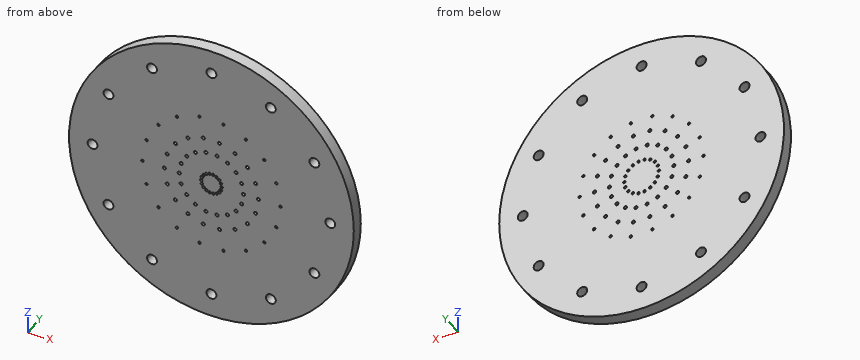
from build123d import *

# Parameters (mm, degrees)
SKETCH1_R           = 73.025
BOSS_EXTRUDE1_DEPTH = 6.35
SKETCH4_R           = 0.59055
CUT_EXTRUDE1_DEPTH  = 50.8475
CUT_EXTRUDE2_START  = -53.3875
SKETCH6_R           = 0.59055
CUT_EXTRUDE2_DEPTH  = 80.524261314
LOX_START           = -7.35
SKETCH7_R           = 0.80645
LOX_HOLES_DEPTH     = 8.35
CIRPATTERN1_COUNT   = 18
SKETCH8_R           = 2.54
CUT_EXTRUDE4_DEPTH  = 7.35
CIRPATTERN2_COUNT   = 12


with BuildPart() as part:
    # Sketch1 → Boss-Extrude1 (new body)
    with BuildSketch(Plane(origin=(0, 0, 0), x_dir=(1, 0, 0), z_dir=(0, 1, 0))):
        Circle(SKETCH1_R)
    extrude(amount=BOSS_EXTRUDE1_DEPTH)

    # Sketch4 → Cut-Extrude1 (cut, through all)
    with BuildSketch(Plane(origin=(-3.917869343, -6.785948759, 0), x_dir=(-0.866025404, 0.5, 0), z_dir=(0.5, 0.866025404, 0))):
        with Locations((-4.52396584, 0)):
            Circle(SKETCH4_R)
    cut_extrude1 = extrude(amount=CUT_EXTRUDE1_DEPTH, mode=Mode.SUBTRACT)

    # Sketch6 → Cut-Extrude2 (cut)
    with BuildSketch(Plane(origin=(5.187869343, -8.985653285, 0), x_dir=(0.866025404, 0.5, 0), z_dir=(0.5, -0.866025404, 0)).offset(CUT_EXTRUDE2_START)):
        with Locations((30.67130657, 0)):
            Circle(SKETCH6_R)
    cut_extrude2 = extrude(amount=CUT_EXTRUDE2_DEPTH, mode=Mode.SUBTRACT)

    # Sketch7 → LOx Holes (cut)
    with BuildSketch(Plane(origin=(0, 6.35, 0), x_dir=(1, 0, 0), z_dir=(0, 1, 0)).offset(LOX_START)):
        with Locations((24.13, 0)):
            Circle(SKETCH7_R)
        with Locations((16.51, 0)):
            Circle(SKETCH7_R)
    lox_holes = extrude(amount=LOX_HOLES_DEPTH, mode=Mode.SUBTRACT)

    # CirPattern1: Cut-Extrude1, Cut-Extrude2, LOx Holes ×18 about axis
    cirpattern1_axis = Axis((0, 0, 0), (0, 1, 0))
    for i in range(1, CIRPATTERN1_COUNT):
        add(cut_extrude1.rotate(cirpattern1_axis, i * 360 / CIRPATTERN1_COUNT), mode=Mode.SUBTRACT)
        add(cut_extrude2.rotate(cirpattern1_axis, i * 360 / CIRPATTERN1_COUNT), mode=Mode.SUBTRACT)
        add(lox_holes.rotate(cirpattern1_axis, i * 360 / CIRPATTERN1_COUNT), mode=Mode.SUBTRACT)

    # Sketch8 → Cut-Extrude4 (cut, through all)
    with BuildSketch(Plane.XZ):
        with Locations((-60.96, 0)):
            Circle(SKETCH8_R)
    cut_extrude4 = extrude(amount=-CUT_EXTRUDE4_DEPTH, mode=Mode.SUBTRACT)

    # CirPattern2: Cut-Extrude4 ×12 about axis
    cirpattern2_axis = Axis((0, 0, 0), (0, 1, 0))
    for i in range(1, CIRPATTERN2_COUNT):
        add(cut_extrude4.rotate(cirpattern2_axis, i * 360 / CIRPATTERN2_COUNT), mode=Mode.SUBTRACT)


solid = part.part
Check sheet for the modelled part. Datum: model origin and axes. Units: mm. Coordinates: 2 decimals unless noted, no trailing zeros. Loops run counter-clockwise (first coordinate to the right, second up) from the corner with the lowest first, then second, coordinate; pieces in that order, holes last. Notation, with made-up numbers: (38, -40) -> (66, -40) arc R9 ccw to (66, -25) -> close; hole circle Ø2 at (-17, 78). An arc over 180 degrees is marked (long way). Write item = value, one per line. Start each with the question number.
1. Section check D-D on x = 47. Record the cut outline in (y, z).
2. Material ranges on line 1 (X direction, y = 6, z = 53); line 2 (Z direction, x = -17.5, y = 0.75); line 3 (X direction, y = 3.75, z = 53.5), recorded low to high.
3. Section check A-A on z = 60.96. Record the cut outline in (x, y).
4. Depth check by flat-ended pin: P1, Ø1, axis at x = 26.5, y = 2, coming from the +Z side; P2, Ø3, axis at y = 1, z = -41.5, coming from the -X side; P3, Ø1, axis at x = 35, y = 5, coming from the +Z side. Enter the tip coordinate at first touch or a pass-through.
5. Section check C-C on y = 1. Give the number of separate pieces and of enclosed holes in the cut face, then the cut area to 3 significant figures.
6. Section check B-B on x = -60.96. Record the cut outline in (y, z).
Responses:
q1.outline = (0, -55.89) -> (6.35, -55.89) -> (6.35, 55.89) -> (0, 55.89) -> close
q2.line_1 = -50.24 to -33.01, -27.95 to 27.95, 33.01 to 50.24
q2.line_2 = -70.9 to -30.95, -29.64 to 29.64, 30.95 to 70.9
q2.line_3 = -49.7 to -32.92, -28.04 to 28.04, 32.92 to 49.7
q3.outline = (-40.21, 0) -> (-2.54, 0) -> (-2.54, 6.35) -> (-40.21, 6.35) -> close; (2.54, 0) -> (40.21, 0) -> (40.21, 6.35) -> (2.54, 6.35) -> close
q4.P1 = 68.24
q4.P2 = -61.1
q4.P3 = 64.36
q5.separate_pieces = 1
q5.enclosed_holes = 84
q5.area = 16,400 mm2
q6.outline = (0, -40.21) -> (6.35, -40.21) -> (6.35, -2.54) -> (0, -2.54) -> close; (0, 2.54) -> (6.35, 2.54) -> (6.35, 40.21) -> (0, 40.21) -> close
